Can you work these out from the model? Positions are in its coordinate system, mm. A direction names the side the tool comes from. Round coordinates to 2 decimals unless told otherwise and drop trailing zeros. Order: outer loops, then holes, each group sorted by start corner. A loop starts at its lowest first (then second) coordinate and runs counter-clockwise, first axis right, second up. Notation, with made-up numbers: (81.25, 27) - (126.25, 27) arc R10 ccw to (126.25, 40) - close; hole circle Ø5 at (83.5, 57). An arc over 180 degrees is marked (long way). Write item = value, one per line.
from build123d import *

# Parameters (mm, degrees)
CROQUIS1_R                   = 25
SALIENTE_EXTRUIR1_DEPTH      = 40
CROQUIS2_R                   = 5
SALIENTE_EXTRUIR2_DEPTH      = 30
REDONDEO1_R                  = 2
CHAFL_N1_SIZE                = 4
SALIENTE_EXTRUIR3_DEPTH      = 2
SALIENTE_EXTRUIR3_DEPTH_BACK = 2
CROQUIS3_R                   = 5
CHAFL_N2_SIZE                = 5


with BuildPart() as part:
    # Croquis1 → Saliente-Extruir1 (new body)
    with BuildSketch(Plane(origin=(0, 0, 0), x_dir=(1, 0, 0), z_dir=(0, 1, 0))):
        with Locations(Location((0, 0, 0), (0, 0, 270))):
            Circle(CROQUIS1_R)
    extrude(amount=SALIENTE_EXTRUIR1_DEPTH)

    # Croquis2 → Saliente-Extruir2 (add)
    with BuildSketch(Plane(origin=(0, 40, 0), x_dir=(1, 0, 0), z_dir=(0, 1, 0))):
        with Locations(Location((0, 0, 0), (0, 0, 270))):
            Circle(CROQUIS2_R)
    extrude(amount=SALIENTE_EXTRUIR2_DEPTH)

    # Redondeo1
    redondeo1_edges = [part.edges().sort_by_distance(p)[0] for p in [
        (0, 70, -5),
    ]]
    fillet(redondeo1_edges, radius=REDONDEO1_R)

    # Chaflán1
    chafl_n1_edges = [part.edges().sort_by_distance(p)[0] for p in [
        (0, 40, -25),
    ]]
    chamfer(chafl_n1_edges, length=CHAFL_N1_SIZE)

    # Croquis3 → Saliente-Extruir3 (add, two sides: drawn at the far end of the back side and taken through both)
    with BuildSketch(Plane.ZY.offset(-25).offset(-SALIENTE_EXTRUIR3_DEPTH_BACK)):
        with Locations((0, 20)):
            Circle(CROQUIS3_R)
    extrude(amount=SALIENTE_EXTRUIR3_DEPTH + SALIENTE_EXTRUIR3_DEPTH_BACK)

    # Redondeo3: read off the stored shape, not the designer's step
    # Redondeo3 outline → Redondeo3 (revolve, cut)
    with BuildSketch(Plane(origin=(0, 20, 0), x_dir=(0, 1, 0), z_dir=(0, 0, -1))):
        with BuildLine():
            Line((5, 27), (3, 27))
            ThreePointArc((3, 27), (4.414213562, 26.414213562), (5, 25))
            Line((5, 25), (5, 27))
        make_face()
    revolve(axis=Axis((0, 20, 0), (1, 0, 0)), mode=Mode.SUBTRACT)

    # Chaflán2
    chafl_n2_edges = [part.edges().sort_by_distance(p)[0] for p in [
        (0, 0, -25),
    ]]
    chamfer(chafl_n2_edges, length=CHAFL_N2_SIZE)


solid = part.part
(1) If we section it at B-B (x = 0): Write out the boundary of the cut face in (y, z), plus the area to 3 significant figures.
Computed:
outline = (0, -20) - (5, -25) - (36, -25) - (40, -21) - (40, -5) - (68, -5) arc R2 ccw to (70, -3) - (70, 3) arc R2 ccw to (68, 5) - (40, 5) - (40, 21) - (36, 25) - (5, 25) - (0, 20) - close
area = 2,260 mm^2
(2) If we section it at A-A (y = 20): Write out the boundary of the cut face in (x, z), plus the area to 3 significant figures.
Computed:
outline = (24.49, -5) - (25, -5) arc R2 ccw to (27, -3) - (27, 3) arc R2 ccw to (25, 5) - (24.49, 5) arc R25 ccw (long way) to start
area = 1,980 mm^2
(3) On a 3-axis mill with a long thin cutter (end or side, diameter ignored), from which of +Z, -Z, +X, -X, +Y, -Y can I reach the whole of each face in a straight line? I mean faces 1 (the face through (6.08, 0.243, 19.308)), 2 (the face through (-4, 40, 4)). Say none if no direction works.
Computed:
face_1 = -Y
face_2 = +Y
(4) If we section it at D-D (y = 44.5): Write out the boundary of the cut face in (x, z), plus the area to 3 significant figures.
Computed:
outline = circle Ø10 at (0, 0)
area = 78.5 mm^2
(5) If I drill on line 1 (X direction, y = 49, z = 0); line 2 (Y direction, x = -8.5, z = -1); line 3 (X direction, y = 36, z = -20.5), over which ranges is the centre line in solid material (lowest first)? Write a range as from..to.
Computed:
line_1 = -5..5
line_2 = 0..40
line_3 = -14.31..14.31
(6) Will these pins go through, and if not, where does the flat tip stop? P1, Ø6, axis at x = 13.5, z = -12.5, coming from the +Y side; P2, Ø12, axis at x = 6.5, y = 59, coming from the +Z side; P3, Ø4, axis at x = 14.5, y = 17.5, coming from the -Z side; P4, Ø2, axis at x = 7, z = 16, coming from the -Y side.
Computed:
P1 = 40
P2 = 4.97
P3 = -21.65
P4 = 0
(7) If we section it at C-C (y = 6.5): Write out the boundary of the cut face in (x, z).
Computed:
outline = circle Ø50 at (0, 0)
